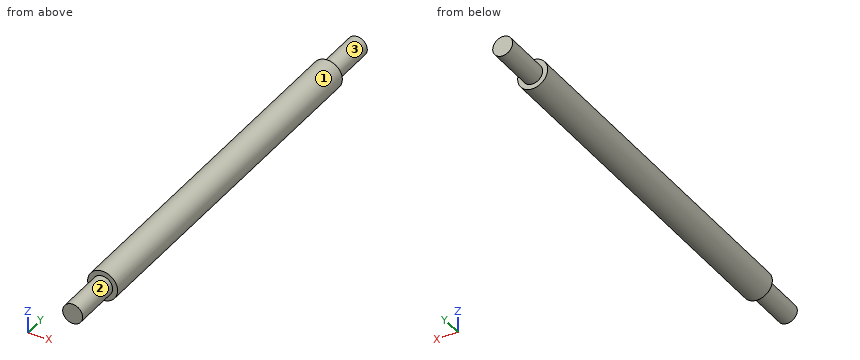
```python
from build123d import *

# Parameters (mm, degrees)
SKETCH1_R           = 3
BOSS_EXTRUDE1_DEPTH = 75
SKETCH2_R           = 2
BOSS_EXTRUDE2_DEPTH = 10
SKETCH3_R           = 2
BOSS_EXTRUDE3_DEPTH = 10


with BuildPart() as part:
    # Sketch1 → Boss-Extrude1 (new body)
    with BuildSketch(Plane(origin=(0, 0, 0), x_dir=(1, 0, 0), z_dir=(0, 1, 0))):
        Circle(SKETCH1_R)
    extrude(amount=BOSS_EXTRUDE1_DEPTH)

    # Sketch2 → Boss-Extrude2 (add)
    with BuildSketch(Plane(origin=(0, 75, 0), x_dir=(1, 0, 0), z_dir=(0, 1, 0))):
        Circle(SKETCH2_R)
    extrude(amount=BOSS_EXTRUDE2_DEPTH)

    # Sketch3 → Boss-Extrude3 (add)
    with BuildSketch(Plane.XZ):
        Circle(SKETCH3_R)
    extrude(amount=BOSS_EXTRUDE3_DEPTH)


solid = part.part
```
The model under review builds one solid part; all positions refer to its coordinate system, in mm. Face numbers are marked on the shaded views. A direction names the side the tool comes from. Give positions to 0.01 mm unless a question says otherwise; leave off trailing zeros. Order: outer loops, then holes, each group sorted by start corner. A loop starts at its lowest first (then second) coordinate and runs counter-clockwise, first axis right, second up. Notation, with made-up numbers: (-19, -4) - (39, -4) arc R28 cw to (39, 28) - close; hole circle Ø6 at (57.25, 81.5). An arc over 180 degrees is marked (long way). Use CSV: the item, a comma, the result in double quotes. Start each with the question number.
Q1. We need section A-A, the plane z = 0. Write out the cut boundary in (x, y), and give its area (3 significant figures).
Q2. We need section D-D, the plane y = 77. Write out the cut boundary in (x, z).
Q3. To check wall thickness, follow line 1 along Y through (x, z) = (0, -2.05); line 2 along X through (y, z) = (44, 1); line 3 along X through (y, z) = (26, 2.15). State the ranges of each line that lie inside material, in increasing order. Write a range as [from, to].
Q4. We need section B-B, the plane x = 0. Write out the cut boundary in (y, z), and give its area (3 significant figures).
Q5. Clearance check with flat-ended pins moving along their axes: pin 1 Ø3 at (y, z) = (39, -2) entering from +X; pin 2 Ø3 at (x, y) = (-1.5, 62.5) entering from -Z. State where each tip first meets the part, or that it passes through.
Q6. We need section C-C, the plane y = 48.5. Write out the cut boundary in (x, z), and give its area (3 significant figures).
Q7. Tool access review of the marked faces 1, 2 and 3: name each direction out of +Z, -Z, +X, -X, +Y, -Y from which nothing blocks a thin tool from reaching the whole face with its end or side.
Outcome:
1,outline,"(-3, 0) - (-2, 0) - (-2, -10) - (2, -10) - (2, 0) - (3, 0) - (3, 75) - (2, 75) - (2, 85) - (-2, 85) - (-2, 75) - (-3, 75) - close"
1,area,"530 mm^2"
2,outline,"circle Ø4 at (0, 0)"
3,line 1,"y = [0, 75]"
3,line 2,"x = [-2.83, 2.83]"
3,line 3,"x = [-2.09, 2.09]"
4,outline,"(-10, -2) - (0, -2) - (0, -3) - (75, -3) - (75, -2) - (85, -2) - (85, 2) - (75, 2) - (75, 3) - (0, 3) - (0, 2) - (-10, 2) - close"
4,area,"530 mm^2"
5,pin 1,"stops at x = 2.96"
5,pin 2,"stops at z = -3"
6,outline,"circle Ø6 at (0, 0)"
6,area,"28.3 mm^2"
7,face 1,"+Y, -Y"
7,face 2,"-Y"
7,face 3,"+Y"
